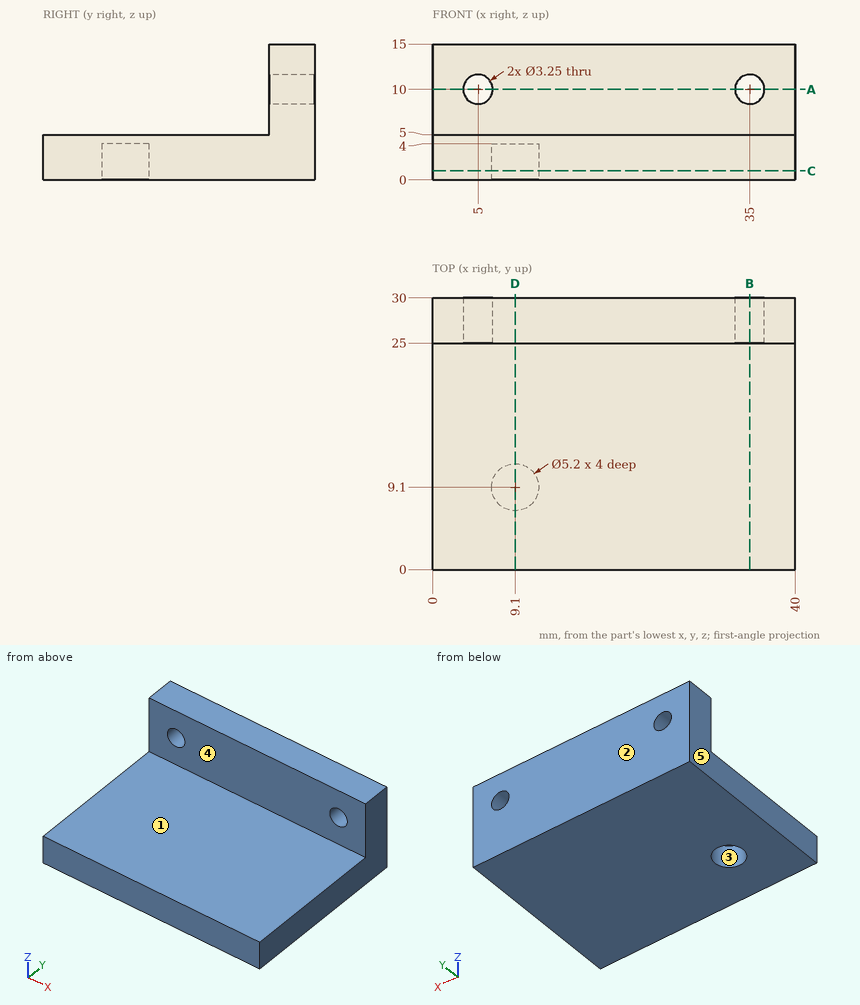
Input: dimensioned drawing with shaded views. Units: mm. Origin: part minimum x, y, z. A direction names the side the tool comes from. Give positions to 0.01 mm unless a question says otherwise; leave off trailing zeros. Loops run counter-clockwise (first coordinate to the right, second up) from the corner with the lowest first, then second, coordinate; pieces in that order, holes last. Notation, with made-up numbers: (-25, 80) -> (27, 80) arc R17 ccw to (27, 113) -> close; hole circle Ø1 at (7, -3.75). An arc over 180 degrees is marked (long way). Use a Markdown table: item, result. Add a question column.
1) First-contact query: pin 1 (5 mm diameter, centred on x = 20, y = 6, fed in from +Z); pin 2 (3 mm diameter, centred on x = 24, z = 9.5, fed in from -Y). Flat tips, straight axial feed; report the tip coordinate or a pass-through.
2) Section query D-D, the plane x = 9.1. Return the cut outline in (y, z), then the cut area to 3 significant figures.
3) Reachability of the marked faces 4 and 5 from +Z, -Z, +X, -X, +Y, -Y: full face, straight path, thin tool, end or side. Return the list, or none.
4) Section query B-B, the plane x = 35. Return the cut outline in (y, z) (3 decimals).
5) Line query: line 1 along Z through (x, y) = (35, 27.75) (3 decimals); line 2 along Y through (x, z) = (9.1, 2.75); line 3 along Y through (x, z) = (34.5, 13.25). Output: solid intervals per line, ascending. Write a range as [from, to].
6) Section query A-A, the plane z = 10. Return the cut outline in (x, y) (3 decimals), then the cut area to 4 significant figures.
7) Pull-direction query (Y, two-part tool) for the marked faces 1, 2 and 3; classes: +Y half, -Y half, draft (parallel to the pull), parting line (faces both ways), or undercut.
8) Section query C-C, the plane z = 1. Return the cut outline in (x, y), then the cut area to 3 significant figures.
Numbers:
| question | item | result |
|---|---|---|
| 1 | pin 1 | stops at z = 5 |
| 1 | pin 2 | stops at y = 25 |
| 2 | outline | (0, 0) -> (6.5, 0) -> (6.5, 4) -> (11.7, 4) -> (11.7, 0) -> (30, 0) -> (30, 15) -> (25, 15) -> (25, 5) -> (0, 5) -> close |
| 2 | area | 179 mm2 |
| 3 | face 4 | +Z, +X, -X, -Y |
| 3 | face 5 | +Z, -Z, -X, +Y, -Y |
| 4 | outline | (0, 0) -> (30, 0) -> (30, 8.375) -> (25, 8.375) -> (25, 5) -> (0, 5) -> close; (25, 11.625) -> (30, 11.625) -> (30, 15) -> (25, 15) -> close |
| 5 | line 1 | z = [0, 8.375], [11.625, 15] |
| 5 | line 2 | y = [0, 6.5], [11.7, 30] |
| 5 | line 3 | y = [25, 30] |
| 6 | outline | (0, 25) -> (3.375, 25) -> (3.375, 30) -> (0, 30) -> close; (6.625, 25) -> (33.375, 25) -> (33.375, 30) -> (6.625, 30) -> close; (36.625, 25) -> (40, 25) -> (40, 30) -> (36.625, 30) -> close |
| 6 | area | 167.5 mm2 |
| 7 | face 1 | draft |
| 7 | face 2 | +Y half |
| 7 | face 3 | undercut |
| 8 | outline | (0, 0) -> (40, 0) -> (40, 30) -> (0, 30) -> close; hole circle Ø5.2 at (9.1, 9.1) |
| 8 | area | 1,180 mm2 |
